```python
from build123d import *

# Parameters (mm, degrees)
SKETCH1_W                      = 27.5
SKETCH1_H                      = 59
SKETCH1_W_2                    = 20.5
SKETCH1_H_2                    = 45
BOSS_EXTRUDE1_DEPTH            = 19.5
CUT_EXTRUDE1_DEPTH             = 39.510550502
CUT_EXTRUDE1_DEPTH_BACK        = 39.510550502
SKETCH2_R                      = 2.25
FILLET1_R                      = 1
SKETCH4_R                      = 4.1
BOSS_EXTRUDE2_DEPTH            = 15.562278481
CBORE_FOR_M3_SHCS1_D           = 3.6
CBORE_FOR_M3_SHCS1_DEPTH       = 5
CBORE_FOR_M3_SHCS1_CBORE_D     = 6.5
CBORE_FOR_M3_SHCS1_CBORE_DEPTH = 3
CUT_EXTRUDE3_REACH             = 57.721
SKETCH5_R                      = 3
CUT_EXTRUDE11_START            = -6.562278481
SKETCH18_R                     = 4.1
SKETCH18_R_2                   = 3.875
CUT_EXTRUDE11_DEPTH            = 6.562278481
CUT_EXTRUDE12_DEPTH            = 56.721269081
CUT_EXTRUDE12_DEPTH_BACK       = 56.721269081
SKETCH20_R                     = 1.5
FILLET10_R                     = 1
CUT_EXTRUDE13_DEPTH            = 69.079165975
CUT_EXTRUDE13_DEPTH_BACK       = 69.079165975
SKETCH21_W                     = 10
SKETCH21_H                     = 15
FILLET8_R                      = 15
CUT_EXTRUDE2_START             = -12
SKETCH3_R                      = 4
CUT_EXTRUDE2_DEPTH             = 33.989141464
FILLET11_R                     = 2
BOSS_EXTRUDE3_START            = 3
SKETCH22_R                     = 1.8
SKETCH22_R_2                   = 3
BOSS_EXTRUDE3_DEPTH            = 3
SKETCH23_R                     = 1.5
CUT_EXTRUDE14_DEPTH            = 52.954182283


# Some blends are built 0.0001 mm under size
with BuildPart() as part:
    # Sketch1 → Boss-Extrude1 (new body)
    with BuildSketch(Plane(origin=(0, 0, 0), x_dir=(1, 0, 0), z_dir=(0, 1, 0))):
        with Locations((1.5, 0)):
            Rectangle(SKETCH1_W, SKETCH1_H)
        Rectangle(SKETCH1_W_2, SKETCH1_H_2, mode=Mode.SUBTRACT)
    extrude(amount=BOSS_EXTRUDE1_DEPTH)

    # Sketch2 → Cut-Extrude1 (cut, two sides: drawn at the far end of the back side and taken through both)
    with BuildSketch(Plane(origin=(0, 19.5, 0), x_dir=(1, 0, 0), z_dir=(0, 1, 0)).offset(-CUT_EXTRUDE1_DEPTH_BACK)):
        with Locations((-5, 24.7)):
            Circle(SKETCH2_R)
        with Locations((5, 24.7)):
            Circle(SKETCH2_R)
        with Locations((5, -24.7)):
            Circle(SKETCH2_R)
        with Locations((-5, -24.7)):
            Circle(SKETCH2_R)
    extrude(amount=CUT_EXTRUDE1_DEPTH + CUT_EXTRUDE1_DEPTH_BACK, mode=Mode.SUBTRACT)

    # Fillet1
    fillet1_edges = [part.edges().sort_by_distance(p)[0] for p in [
        (5.471699057, 9.75, 22.5),
        (4.528300943, 9.75, 22.5),
        (-4.528300943, 9.75, 22.5),
        (-5.471699057, 9.75, 22.5),
        (-5.471699057, 9.75, -22.5),
        (-4.528300943, 9.75, -22.5),
        (4.528300943, 9.75, -22.5),
        (5.471699057, 9.75, -22.5),
    ]]
    fillet(fillet1_edges, radius=FILLET1_R)

    # Sketch4 → Boss-Extrude2 (add)
    with BuildSketch(Plane.ZY.offset(12.25)):
        with Locations(Location((0, 15.4, 0), (0, 0, 90))):
            Circle(SKETCH4_R)
    extrude(amount=BOSS_EXTRUDE2_DEPTH)

    # CBORE for M3 SHCS1
    with Locations(Plane.ZY.offset(-10.25)):
        with Locations((-7, 15.4), (7, 15.4), (0, 8.4)):
            CounterBoreHole(CBORE_FOR_M3_SHCS1_D / 2, CBORE_FOR_M3_SHCS1_CBORE_D / 2, CBORE_FOR_M3_SHCS1_CBORE_DEPTH, depth=CBORE_FOR_M3_SHCS1_DEPTH)

    # Sketch5 → Cut-Extrude3 (cut, up to next)
    with BuildSketch(Plane(origin=(15.25, 0, 0), x_dir=(0, 0, -1), z_dir=(1, 0, 0)), mode=Mode.PRIVATE) as cut_extrude3_sk1:
        with Locations((0, 15.4)):
            Circle(SKETCH5_R)
    cut_extrude3_tool1 = extrude(cut_extrude3_sk1.sketch, amount=-CUT_EXTRUDE3_REACH, mode=Mode.PRIVATE) & part.part
    add(cut_extrude3_tool1.solids().sort_by_distance((15.25, 15.4, 0))[0], mode=Mode.SUBTRACT)

    # Sketch18 → Cut-Extrude11 (cut)
    with BuildSketch(Plane.ZY.offset(27.812278481).offset(CUT_EXTRUDE11_START)):
        with Locations(Location((0, 15.4, 0), (0, 0, 180))):
            Circle(SKETCH18_R)
        with Locations(Location((0, 15.4, 0), (0, 0, 270))):
            Circle(SKETCH18_R_2, mode=Mode.SUBTRACT)
    extrude(amount=CUT_EXTRUDE11_DEPTH, mode=Mode.SUBTRACT)

    # Sketch20 → Cut-Extrude12 (cut, two sides: drawn at the far end of the back side and taken through both)
    with BuildSketch(Plane.ZY.offset(27.812278481).offset(-CUT_EXTRUDE12_DEPTH_BACK)):
        with Locations(Location((0, 15.4, 0), (0, 0, 180))):
            Circle(SKETCH20_R)
    extrude(amount=CUT_EXTRUDE12_DEPTH + CUT_EXTRUDE12_DEPTH_BACK, mode=Mode.SUBTRACT)

    # Fillet10
    fillet10_edges = [part.edges().sort_by_distance(p)[0] for p in [
        (-27.812278481, 19.275, 0),
    ]]
    fillet(fillet10_edges, radius=FILLET10_R)

    # Sketch21 → Cut-Extrude13 (cut, two sides: drawn at the far end of the back side and taken through both)
    with BuildSketch(Plane(origin=(0, 0, -29.5), x_dir=(-1, 0, 0), z_dir=(0, 0, -1)).offset(-CUT_EXTRUDE13_DEPTH_BACK)):
        Rectangle(SKETCH21_W, SKETCH21_H)
    extrude(amount=CUT_EXTRUDE13_DEPTH + CUT_EXTRUDE13_DEPTH_BACK, mode=Mode.SUBTRACT)

    # Fillet8
    # the kernel refuses this fillet: 15 mm, written as the material it takes off along each edge
    with BuildSketch(Plane(origin=(-49.75, 0, 29.5), x_dir=(0, 0, -1), z_dir=(1, 0, 0)), Plane(origin=(32.5, 0, -29.5), x_dir=(0, 0, 1), z_dir=(-1, 0, 0))) as fillet8_piece_1:
        with BuildLine():
            CenterArc((FILLET8_R, FILLET8_R), FILLET8_R, 180, 90)
            Line((0, FILLET8_R), (0, 0))
            Line((0, 0), (FILLET8_R, 0))
        make_face()
    extrude(amount=82.25, mode=Mode.SUBTRACT)
    with BuildSketch(Plane(origin=(-32.5, 0, 29.5), x_dir=(0, 1, 0), z_dir=(1, 0, 0)), Plane(origin=(52.75, 0, -29.5), x_dir=(0, 1, 0), z_dir=(-1, 0, 0))) as fillet8_piece_2:
        with BuildLine():
            CenterArc((FILLET8_R, -FILLET8_R), FILLET8_R, 90, 90)
            Line((0, -FILLET8_R), (0, 0))
            Line((0, 0), (FILLET8_R, 0))
        make_face()
    extrude(amount=85.25, mode=Mode.SUBTRACT)

    # Sketch3 → Cut-Extrude2 (cut, through all)
    with BuildSketch(Plane(origin=(0, 19.5, 0), x_dir=(1, 0, 0), z_dir=(0, 1, 0)).offset(CUT_EXTRUDE2_START)):
        with Locations((-5, -24.7)):
            Circle(SKETCH3_R)
        with Locations((5, -24.7)):
            Circle(SKETCH3_R)
        with Locations((5, 24.7)):
            Circle(SKETCH3_R)
        with Locations((-5, 24.7)):
            Circle(SKETCH3_R)
    extrude(amount=-CUT_EXTRUDE2_DEPTH, mode=Mode.SUBTRACT)

    # Fillet11
    fillet11_edges = [part.edges().sort_by_distance(p)[0] for p in [
        (-12.25, 0, 0),
        (-12.25, 4.393398282, 25.106601718),
        (-12.25, 4.393398282, -25.106601718),
        (15.25, 0, 0),
        (15.25, 4.393398282, -25.106601718),
        (15.25, 4.393398282, 25.106601718),
        (15.25, 17.25, 29.5),
        (-12.25, 17.25, 29.5),
        (-12.25, 17.25, -29.5),
        (15.25, 17.25, -29.5),
    ]]
    fillet(fillet11_edges, radius=FILLET11_R - 0.0001)  # a hair under: the kernel refuses the full size

    # Sketch22 → Boss-Extrude3 (add)
    with BuildSketch(Plane(origin=(15.25, 0, 0), x_dir=(0, 0, -1), z_dir=(1, 0, 0)).offset(BOSS_EXTRUDE3_START)):
        with BuildLine():
            Line((9.120855223, 19.5), (-9.120855223, 19.5))
            ThreePointArc((-9.120855223, 19.5), (0, 5.4), (9.120855223, 19.5))
        make_face()
        with Locations(Location((7, 15.4, 0), (0, 0, 180))):
            Circle(SKETCH22_R, mode=Mode.SUBTRACT)
        with Locations(Location((0, 8.4, 0), (0, 0, 180))):
            Circle(SKETCH22_R, mode=Mode.SUBTRACT)
        with Locations((0, 15.4)):
            Circle(SKETCH22_R_2, mode=Mode.SUBTRACT)
        with Locations(Location((-7, 15.4, 0), (0, 0, 180))):
            Circle(SKETCH22_R, mode=Mode.SUBTRACT)
    extrude(amount=-BOSS_EXTRUDE3_DEPTH)

    # Sketch23 → Cut-Extrude14 (cut, through all)
    with BuildSketch(Plane.ZY.offset(-10.25)):
        with Locations(Location((0, 8.4, 0), (0, 0, 180))):
            Circle(SKETCH23_R)
    extrude(amount=CUT_EXTRUDE14_DEPTH, mode=Mode.SUBTRACT)


solid = part.part
```
Geometry: final body of the model. Coordinates: model frame, mm. A direction names the side the tool comes from. Round coordinates to 2 decimals unless told otherwise and drop trailing zeros. Write each loop counter-clockwise with the first axis right and the second up, starting at its lowest first coordinate (ties: lowest second). Pieces come first, ordered by that corner, then holes. Notation, with made-up numbers: (61, -7) -> (69, -7) arc R15 ccw to (69, 15) -> close; hole circle Ø5 at (7, -12). An arc over 180 degrees is marked (long way). Return JSON: item names as keys, results as strings.
Q1. Section A-A on z = -7. Give the number of separate pieces and of enclosed holes in the cut face, and give its area (3 significant figures).
From the geometry:
{"separate pieces": "3", "enclosed holes": "0", "area": "131 mm2"}
Q2. Section B-B on x = -14. Return the cut outline in (y, z), and give its area (3 significant figures).
From the geometry:
{"outline": "circle Ø8.2 at (15.4, 0); hole circle Ø3 at (15.4, 0)", "area": "45.7 mm2"}
Q3. Mould query, pull axis X, two halves, no side actions, for faces 5 (the cylindrical face through (-8.99, 5.52, 24.44)), 6 (the flat face through (-27.812, 17, 1)), 7 (the flat face through (0, 7.5, 25)), 8 (the cylindrical face through (14.68, 17.28, -28.9)). Classes: +X half, -X half, draft (parallel to the pull), parting line (faces both ways), or undercut.
From the geometry:
{"face 5": "undercut", "face 6": "-X half", "face 7": "undercut", "face 8": "+X half"}
Q4. First-contact query: pin 1 Ø5 at (y, z) = (15.4, -7) entering from +X; pin 2 Ø1.5 at (x, y) = (-21, 16.5) entering from -Z; pin 3 Ø2 at (y, z) = (7, -1.5) entering from -X; pin 4 Ø0.7 at (x, y) = (-9, 10) entering from -Z. Flat tips, straight axial feed; report the tip coordinate or a pass-through.
From the geometry:
{"pin 1": "x = 18.25", "pin 2": "z = -4.09", "pin 3": "x = -12.25", "pin 4": "z = -28.76"}
Q5. Ray query, line 1 (X direction, y = 13.5, z = -24.7); line 2 (Y direction, x = 12.4, z = 7); line 3 (X direction, y = 7.5, z = 2). Return the intervals inside material, ascending.
From the geometry:
{"line 1": "-12.25 to -7.25, -2.75 to 2.75, 7.25 to 15.25", "line 2": "0 to 12.15, 18.65 to 19.5", "line 3": "-12.25 to -10.25, 13.25 to 18.25"}
Q6. Set-up query: faces 1 (the flat face through (13.25, 14, 8.4)), 2 (the flat face through (-9, 11, 22.5)), 3 (the cylindrical face through (4.276, 8.811, -28.163)), 4 (the cylindrical face through (8.99, 5.52, -24.44)). Return all of +Z, -Z, +X, -X, +Y, -Y with unobstructed straight access to the full face (end or side cutting, diameter ignored); none if empty.
From the geometry:
{"face 1": "none", "face 2": "+Y, -Y", "face 3": "-Z, +X, -X, -Y", "face 4": "-Y"}
